```python
from build123d import *
from OCP.BRepFilletAPI import BRepFilletAPI_MakeChamfer

# Parameters (mm, degrees)
CROQUIS1_W              = 85
CROQUIS1_H              = 30
CROQUIS1_W_2            = 16
CROQUIS1_H_2            = 23
SALIENTE_EXTRUIR1_DEPTH = 3
CROQUIS3_W              = 37
CROQUIS3_H              = 30
SALIENTE_EXTRUIR2_DEPTH = 10
CHAFL_N1_SIZE           = 10
CHAFL_N1_SIZE_2         = 8.390996312


with BuildPart() as part:
    # Croquis1 → Saliente-Extruir1 (new body)
    with BuildSketch(Plane(origin=(0, 0, 0), x_dir=(1, 0, 0), z_dir=(0, 1, 0))):
        Rectangle(CROQUIS1_W, CROQUIS1_H)
        with Locations((30, 0)):
            Rectangle(CROQUIS1_W_2, CROQUIS1_H_2, mode=Mode.SUBTRACT)
        with Locations((-30, 0)):
            Rectangle(CROQUIS1_W_2, CROQUIS1_H_2, mode=Mode.SUBTRACT)
    extrude(amount=SALIENTE_EXTRUIR1_DEPTH)

    # Croquis3 → Saliente-Extruir2 (add)
    with BuildSketch(Plane(origin=(0, 3, 0), x_dir=(1, 0, 0), z_dir=(0, 1, 0))):
        Rectangle(CROQUIS3_W, CROQUIS3_H)
    extrude(amount=SALIENTE_EXTRUIR2_DEPTH)

    # Chaflán1
    chafl_n1_edges_1 = [part.edges().sort_by_distance(p)[0] for p in [
        (18.5, 13, 0),
    ]]
    chafl_n1_side_1 = [part.faces().sort_by_distance(p)[0] for p in [
        (18.5, 12.832180074, 0),
    ]]
    chafl_n1_edges_2 = [part.edges().sort_by_distance(p)[0] for p in [
        (-18.5, 13, 0),
    ]]
    chafl_n1_side_2 = [part.faces().sort_by_distance(p)[0] for p in [
        (-18.5, 12.832180074, 0),
    ]]
    chafl_n1 = BRepFilletAPI_MakeChamfer(part.part.solid().wrapped)
    for e in chafl_n1_edges_1:
        chafl_n1.Add(CHAFL_N1_SIZE - 0.0001, CHAFL_N1_SIZE_2 - 0.0001, e.wrapped, chafl_n1_side_1[0].wrapped)
    for e in chafl_n1_edges_2:
        chafl_n1.Add(CHAFL_N1_SIZE - 0.0001, CHAFL_N1_SIZE_2 - 0.0001, e.wrapped, chafl_n1_side_2[0].wrapped)
    add(Compound.cast(chafl_n1.Shape()), mode=Mode.REPLACE)  # a hair under: the kernel refuses the full size


solid = part.part
```
Geometry: final body of the model. Coordinates: model frame, mm. A direction names the side the tool comes from. Coordinates: 2 decimals unless noted, no trailing zeros. Order: outer loops, then holes, each group sorted by start corner. A loop starts at its lowest first (then second) coordinate and runs counter-clockwise, first axis right, second up. Notation, with made-up numbers: M 39,-30.75 L 88,-30.75 A20 cw 88,-25.75 Z; hole C 39.25,51.25 d11. An arc over 180 degrees is marked long. Answer as CSV lines item,"result".
Q1. First-contact query: P1, Ø7, axis at x = -25, z = -6, coming from the +Y side; P2, Ø4, axis at y = 6.5, z = 11.5, coming from the +X side; P3, Ø1.5, axis at y = 11, z = -3, coming from the -X side. Flat tips, straight axial feed; report the tip coordinate or a pass-through.
Answers:
P1,"stops at y = 3"
P2,"stops at x = 17.24"
P3,"stops at x = -12.42"
Q2. Section D-D on x = 20. Return the cut outline in (y, z).
Answers:
outline,"M 0,-15 L 3,-15 L 3,15 L 0,15 Z"
Q3. Set-up query: faces 4 (the flat face through (-39, 3, 0)), 5 (the flat face through (-30, 1, -11.5)), 6 (the flat face through (38.3, 3, -0.2)). Return all of +Z, -Z, +X, -X, +Y, -Y with unobstructed straight access to the full face (end or side cutting, diameter ignored); none if empty.
Answers:
face 4,"+Z, -Z, -X, +Y"
face 5,"+Y, -Y"
face 6,"+Z, -Z, +X, +Y"
Q4. Line query: probe 1 along X at (y, z) = (1.5, 1.5); probe 2 along Z at (x, y) = (22.5, 2); probe 3 along Y at (x, z) = (20, -7). Output: solid intervals per line, ascending. Write a range as [from, to].
Answers:
probe 1,"x = [-42.5, -38], [-22, 22], [38, 42.5]"
probe 2,"z = [-15, -11.5], [11.5, 15]"
probe 3,"y = [0, 3]"
Q5. Draft query along X for faces 1 (the flat face through (-42.5, 1, 0)), 2 (the flat face through (30, 1, 11.5)), 3 (the flat face through (-1, 0, 0)). Return one class per face: pulls with the +X half, pulls with the -X half, needs draft (parallel to the pull), parting line crosses it, or undercut.
Answers:
face 1,"pulls with the -X half"
face 2,"undercut"
face 3,"needs draft"
Q6. Section A-A on x = -33. Return the cut outline in (y, z).
Answers:
outline,"M 0,-15 L 3,-15 L 3,-11.5 L 0,-11.5 Z; M 0,11.5 L 3,11.5 L 3,15 L 0,15 Z"
Q7. Section C-C on y = 11. Return the cut outline in (x, z).
Answers:
outline,"M -11.79,-15 L 11.79,-15 L 11.79,15 L -11.79,15 Z"
Q8. Section B-B on z = -7. Count the separate pieces of the cut face and the enclosed holes in it, and give its area (3 significant figures).
Answers:
separate pieces,"3"
enclosed holes,"0"
area,"445 mm^2"
